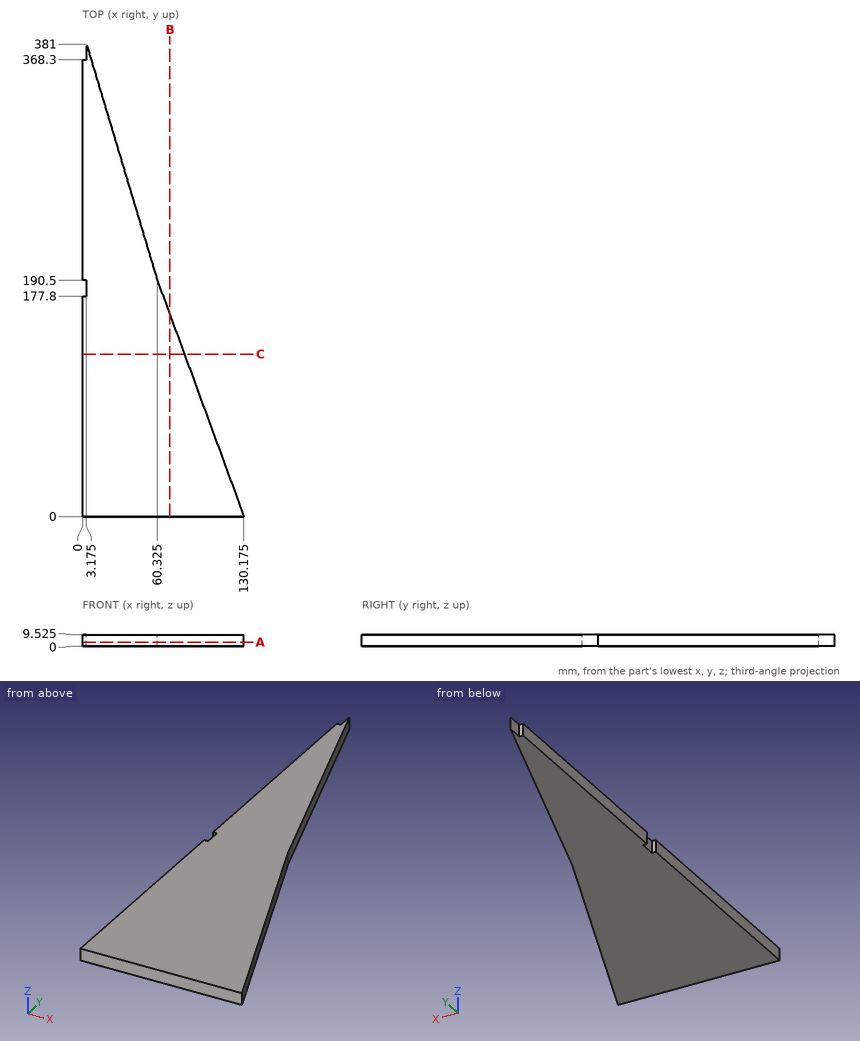
Study the drawing (mm; zero at the part's minimum x, y, z) and answer. Give positions to 0.01 mm unless a question says otherwise; leave off trailing zeros. Order: outer loops, then holes, each group sorted by start corner. A loop starts at its lowest first (then second) coordinate and runs counter-clockwise, first axis right, second up. Notation, with made-up numbers: M 86.5,55 L 92.5,55 A27 cw 92.5,73 Z; hole C 62,76 d7. An arc over 180 degrees is marked long. Put each result on its own line as item: value. Start each with the question number.
Item 1: The part is cut by section C-C, the plane y = 131. Determine the outline of the cut face in (x, z) (3 decimals).
Item 2: Flat-ended cylindrical pins translate along their axes: P1, Ø3, axis at y = 376, z = 3, coming from the -X side (3 decimals); P2, Ø1.6, axis at x = 1, z = 6, coming from the +Y side. Find the tip coordinate at first contact, or state that the pin passes through.
Item 3: Find the intervals of material crossed by line 1 along X through (y, z) = (289, 8.75) (3 decimals); line 2 along X through (y, z) = (296.5, 7.75) (3 decimals), in increasing order.
Item 4: The part is cut by section A-A, the plane z = 3.5. Determine the outline of the cut face in (x, y) (3 decimals).
Item 5: The part is cut by section B-B, the plane x = 70.5. Determine the outline of the cut face in (y, z) (3 decimals).
Answer key:
1. outline: M 0,0 L 82.142,0 L 82.142,9.525 L 0,9.525 Z
2. P1: stops at x = 3.175
2. P2: stops at y = 368.3
3. line 1: x = 0 to 30.775
3. line 2: x = 0 to 28.525
4. outline: M 0,0 L 130.175,0 L 60.325,190.5 L 3.175,381 L 3.175,368.3 L 0,368.3 L 0,190.5 L 3.175,190.5 L 3.175,177.8 L 0,177.8 Z
5. outline: M 0,0 L 162.75,0 L 162.75,9.525 L 0,9.525 Z
